Print and shaded views of the part. All mm, measured from the part's lowest x, y and z. Round coordinates to 2 decimals unless told otherwise and drop trailing zeros. Order: outer loops, then holes, each group sorted by start corner. A loop starts at its lowest first (then second) coordinate and runs counter-clockwise, first axis right, second up. Notation, with made-up numbers: (71, 41.25) - (114, 41.25) arc R21 ccw to (114, 75.25) - close; hole circle Ø8 at (81.5, -19.75). An arc over 180 degrees is marked (long way). Return JSON: item names as keys, results as strings. Group by question number.
Item 1: Two-plate mould, pull along Y, no slides. Class the marked faces 1, 2, 3 and 4: released by +Y, released by -Y, zero draft, split by the parting line, or undercut.
Item 2: Saw through at C-C on z = 38. List the corners of the cut face in (x, y) (1 decimal), and give its area (3 significant figures).
Item 3: Saw through at B-B on y = 2.5. List the corners of the cut face in (x, z), and give its area (3 significant figures).
Item 4: Probe probe 1 along X at (y, z) = (9.5, 19); probe 2 along X at (y, z) = (9.5, 36); probe 3 along Y at (x, z) = (7, 16). List the from-to ranges inside material, lowest first.
Item 5: Drop flat-ended pins along their axis: pin 1 (8 mm diameter, centred on x = 11.5, z = 12, fed in from -Y); pin 2 (2 mm diameter, centred on x = 4, z = 13.5, fed in from -Y); pin 3 (5 mm diameter, centred on x = 13, z = 33.5, fed in from +Y). Give the stop position or say it passes through.
Item 6: Saw through at A-A on z = 27.5. List the corners of the cut face in (x, y) (1 decimal).
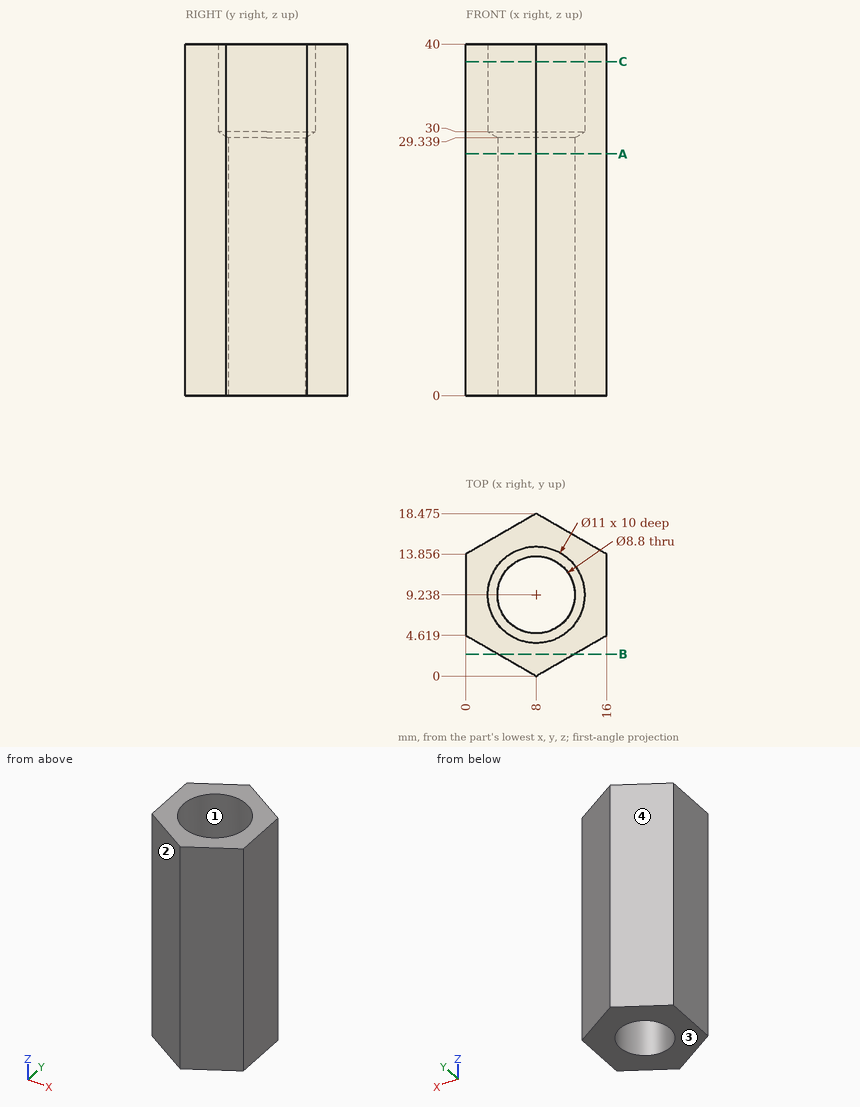
Filled in:
{
 "1": {"face 1": "undercut", "face 2": "released by -Y", "face 3": "zero draft", "face 4": "released by +Y"},
 "2": {"outline": "(0, 4.6) - (8, 0) - (16, 4.6) - (16, 13.9) - (8, 18.5) - (0, 13.9) - close; hole circle Ø11 at (8, 9.2)", "area": "127 mm^2"},
 "3": {"outline": "(3.67, 0) - (12.33, 0) - (12.33, 40) - (3.67, 40) - close", "area": "346 mm^2"},
 "4": {"probe 1": "x = 0 to 3.61, 12.39 to 16", "probe 2": "x = 0 to 2.51, 13.49 to 16", "probe 3": "y = 0.58 to 4.95, 13.52 to 17.9"},
 "5": {"pin 1": "stops at y = 0", "pin 2": "stops at y = 1.73", "pin 3": "stops at y = 17.03"},
 "6": {"outline": "(0, 4.6) - (8, 0) - (16, 4.6) - (16, 13.9) - (8, 18.5) - (0, 13.9) - close; hole circle Ø8.8 at (8, 9.2)"}
}
